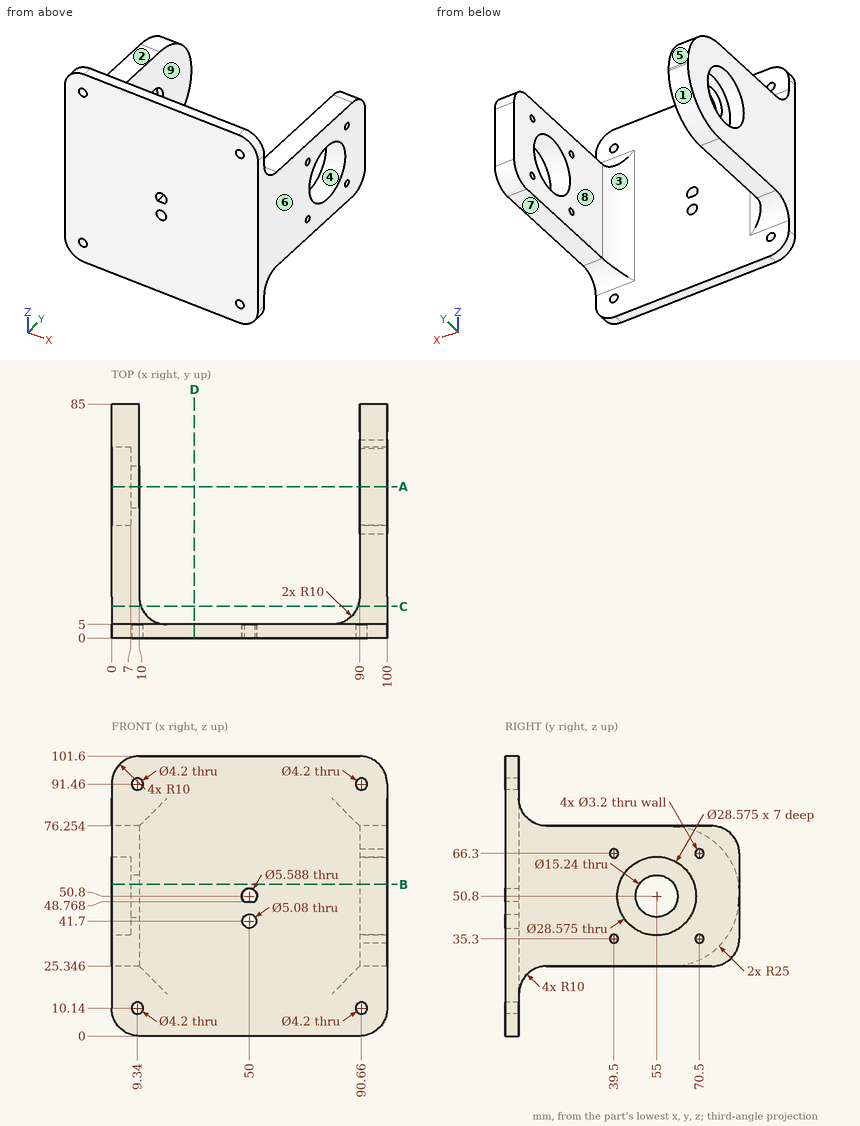
Check sheet for the drawn part. Datum: minimum x, y, z corner. Units: mm. A direction names the side the tool comes from. Round coordinates to 2 decimals unless told otherwise and drop trailing zeros. Order: outer loops, then holes, each group sorted by start corner. A loop starts at its lowest first (then second) coordinate and runs counter-clockwise, first axis right, second up. Notation, with made-up numbers: (12, -16) - (32, -16) arc R10 ccw to (32, -2) - close; hole circle Ø6 at (57.5, 36.5). An arc over 180 degrees is marked (long way). Use a Markdown table: item, result. Add a question column.
(1) Sectioned sample at D-D, the plane x = 30. Enter the section's corners in (y, z).
(2) Material ranges on line 1 along Z through (x, y) = (9.34, 2.95); line 2 along Z through (x, y) = (50, 1.75); line 3 along X through (y, z) = (54, 72.5), recorded low to high. Write a range as [from, to].
(3) Release check for a two-part mould opening along X. For the marked faces 6, 7, 8 and 9 record: pulls with the +X half, pulls with the -X half, needs draft (parallel to the pull), parting line crosses it, or undercut.
(4) Sectioned sample at A-A, the plane y = 55. Enter the section's corners in (x, z), and give its area (3 significant figures).
(5) Sectioned sample at C-C, the plane y = 11.5. Enter the section's corners in (x, z), and give its area (3 significant figures).
(6) Depth check by flat-ended pin: pin 1 (2 mm diameter, centred on y = 25.5, z = 38.5, fed in from -X); pin 2 (12 mm diameter, centred on y = 55, z = 50.8, fed in from -X); pin 3 (5 mm diameter, centred on x = 77, z = 84.5, fed in from +Y); pin 4 (15.5 mm diameter, centred on y = 58.5, z = 53.5, fed in from +X). Enter the tip coordinate at first touch or a pass-through.
(7) Tool access check on the marked faces 1, 2, 3, 4 and 5. Record the directions out of +Z, -Z, +X, -X, +Y, -Y that give a thin tool (end or side, any length) a straight path to the whole face; none if there is none.
(8) Sectioned sample at B-B, the plane z = 55. Enter the section's corners in (x, y), and give its area (3 significant figures).
Answers below:
| question | item | result |
|---|---|---|
| 1 | outline | (0, 0) - (5, 0) - (5, 101.6) - (0, 101.6) - close |
| 2 | line 1 | [0.02, 8.04], [12.24, 89.36], [93.56, 101.58] |
| 2 | line 2 | [0, 39.16], [44.24, 48.77], [53.59, 101.6] |
| 2 | line 3 | [0, 10], [90, 100] |
| 3 | face 6 | pulls with the +X half |
| 3 | face 7 | needs draft |
| 3 | face 8 | undercut |
| 3 | face 9 | undercut |
| 4 | outline | (0, 25.35) - (10, 25.35) - (10, 43.18) - (7, 43.18) - (7, 36.51) - (0, 36.51) - close; (0, 65.09) - (7, 65.09) - (7, 58.42) - (10, 58.42) - (10, 76.25) - (0, 76.25) - close; (90, 25.35) - (100, 25.35) - (100, 36.51) - (90, 36.51) - close; (90, 65.09) - (100, 65.09) - (100, 76.25) - (90, 76.25) - close |
| 4 | area | 487 mm² |
| 5 | outline | (0, 24.71) - (10.63, 24.71) - (10.63, 76.89) - (0, 76.89) - close; (89.37, 24.71) - (100, 24.71) - (100, 76.89) - (89.37, 76.89) - close |
| 5 | area | 1,110 mm² |
| 6 | pin 1 | x = 0 |
| 6 | pin 2 | through |
| 6 | pin 3 | y = 5 |
| 6 | pin 4 | x = 10 |
| 7 | face 1 | -Z, -X, +Y |
| 7 | face 2 | +Z, +X, -X, +Y |
| 7 | face 3 | +Z, -Z, +Y |
| 7 | face 4 | +X |
| 7 | face 5 | +Z, -X, +Y |
| 8 | outline | (0, 0) - (100, 0) - (100, 41.34) - (90, 41.34) - (90, 15) arc R10 cw to (80, 5) - (20, 5) arc R10 cw to (10, 15) - (10, 48.64) - (7, 48.64) - (7, 41.34) - (0, 41.34) - close; (0, 68.66) - (7, 68.66) - (7, 61.36) - (10, 61.36) - (10, 84.72) - (0, 84.72) - close; (90, 68.66) - (100, 68.66) - (100, 85) - (90, 85) - close |
| 8 | area | 1,640 mm² |
